```python
from build123d import *

# Parameters (mm, degrees)
SCHIZZO2_W                   = 111.2
SCHIZZO2_H                   = 55
ESTRUSIONE_ESTRUSIONE1_DEPTH = 15
SCHIZZO3_W                   = 14.8
SCHIZZO3_H                   = 55
ESTRUSIONE_ESTRUSIONE2_DEPTH = 24
SCHIZZO4_W                   = 55
SCHIZZO4_H                   = 11.8
ESTRUSIONE_ESTRUSIONE3_DEPTH = 10
SMUSSO1_SIZE                 = 5
SMUSSO2_SIZE                 = 5
FORO_6_0_6_1_D               = 6
SPECCHIA11_COPY_1_D          = 6
SCHIZZO10_R                  = 5.5
TAGLIO_ESTRUSIONE3_DEPTH     = 9
SPECCHIA13_COPY_1_SKETCH_R   = 5.5
SPECCHIA13_COPY_1_DEPTH      = 9
RACCORDO1_R                  = 2
CUT_EXTRUDE1_REACH           = 123.007
SKETCH2_W                    = 27.5
SKETCH2_H                    = 6
SKETCH3_W                    = 111.2
SKETCH3_H                    = 39
BOSS_EXTRUDE1_DEPTH          = 5
SKETCH5_R                    = 15.6
BOSS_EXTRUDE2_DEPTH          = 5.9
FILLET1_R                    = 1
FILLET2_R                    = 5
SCHIZZO11_R                  = 2.9
ESTRUSIONE_ESTRUSIONE4_DEPTH = 5.9
RACCORDO2_R                  = 1
CUT_EXTRUDE2_REACH           = 124.24
SKETCH6_R                    = 2.5
CUT_EXTRUDE3_REACH           = 124.24
SKETCH7_R                    = 2.5
SKETCH8_R                    = 4.5
CUT_EXTRUDE4_DEPTH           = 5
SKETCH9_R                    = 4.5
CUT_EXTRUDE5_DEPTH           = 5


with BuildPart() as part:
    # Schizzo2 → Estrusione-Estrusione1 (new body)
    with BuildSketch(Plane(origin=(0, 0, 0), x_dir=(1, 0, 0), z_dir=(0, 1, 0))):
        Rectangle(SCHIZZO2_W, SCHIZZO2_H)
    extrude(amount=ESTRUSIONE_ESTRUSIONE1_DEPTH)

    # Schizzo3 → Estrusione-Estrusione2 (add)
    with BuildSketch(Plane(origin=(0, 15, 0), x_dir=(1, 0, 0), z_dir=(0, 1, 0))):
        with Locations((48.2, 0)):
            Rectangle(SCHIZZO3_W, SCHIZZO3_H)
    estrusione_estrusione2 = extrude(amount=ESTRUSIONE_ESTRUSIONE2_DEPTH)

    # Schizzo4 → Estrusione-Estrusione3 (add)
    with BuildSketch(Plane.ZY.offset(-40.8)):
        with Locations((0, 33.1)):
            Rectangle(SCHIZZO4_W, SCHIZZO4_H)
    estrusione_estrusione3 = extrude(amount=ESTRUSIONE_ESTRUSIONE3_DEPTH)

    # Smusso1
    smusso1_edges = [part.edges().sort_by_distance(p)[0] for p in [
        (30.8, 33.1, 27.5),
    ]]
    chamfer(smusso1_edges, length=SMUSSO1_SIZE)

    # Specchia2: Estrusione-Estrusione2 across plane
    add(estrusione_estrusione2.mirror(Plane(origin=(0, 0, 0), x_dir=(0, 0, 1), z_dir=(1, 0, 0))))

    # Specchia3: Estrusione-Estrusione3 across plane
    add(estrusione_estrusione3.mirror(Plane(origin=(0, 0, 0), x_dir=(0, 0, 1), z_dir=(1, 0, 0))))

    # Smusso2
    smusso2_edges = [part.edges().sort_by_distance(p)[0] for p in [
        (-30.8, 33.1, 27.5),
    ]]
    chamfer(smusso2_edges, length=SMUSSO2_SIZE)

    # Foro Ø6.0 (6)-1 (through all)
    with Locations(Plane(origin=(0, 15, 0), x_dir=(1, 0, 0), z_dir=(0, 1, 0))):
        with Locations((17.67766953, 17.67766953)):
            foro_6_0_6_1 = Hole(FORO_6_0_6_1_D / 2)

    # Specchia10: Foro Ø6.0 (6)-1 across plane
    add(foro_6_0_6_1.mirror(Plane.XY), mode=Mode.SUBTRACT)

    # Specchia11: Foro Ø6.0 (6)-1 across plane
    add(foro_6_0_6_1.mirror(Plane(origin=(0, 0, 0), x_dir=(0, 0, 1), z_dir=(1, 0, 0))), mode=Mode.SUBTRACT)

    # Specchia11 copy 1 (through all)
    with Locations(Plane(origin=(0, 15, 0), x_dir=(-1, 0, 0), z_dir=(0, 1, 0))):
        with Locations((17.67766953, 17.67766953)):
            Hole(SPECCHIA11_COPY_1_D / 2)

    # Schizzo10 → Taglio-Estrusione3 (cut)
    with BuildSketch(Plane(origin=(0, 15, 0), x_dir=(1, 0, 0), z_dir=(0, 1, 0))):
        with Locations(Location((17.67766953, 17.67766953, 0), (0, 0, 270))):
            Circle(SCHIZZO10_R)
    taglio_estrusione3 = extrude(amount=-TAGLIO_ESTRUSIONE3_DEPTH, mode=Mode.SUBTRACT)

    # Specchia12: Taglio-Estrusione3 across plane
    add(taglio_estrusione3.mirror(Plane.XY), mode=Mode.SUBTRACT)

    # Specchia13: Taglio-Estrusione3 across plane
    add(taglio_estrusione3.mirror(Plane(origin=(0, 0, 0), x_dir=(0, 0, 1), z_dir=(1, 0, 0))), mode=Mode.SUBTRACT)

    # Specchia13 copy 1 sketch → Specchia13 copy 1 (cut)
    with BuildSketch(Plane(origin=(0, 15, 0), x_dir=(-1, 0, 0), z_dir=(0, 1, 0))):
        with Locations(Location((17.67766953, 17.67766953, 0), (0, 0, 270))):
            Circle(SPECCHIA13_COPY_1_SKETCH_R)
    extrude(amount=-SPECCHIA13_COPY_1_DEPTH, mode=Mode.SUBTRACT)

    # Raccordo1
    raccordo1_edges = [part.edges().sort_by_distance(p)[0] for p in [
        (30.8, 27.2, -2.5),
        (30.8, 39, -2.5),
        (-30.8, 27.2, -2.5),
        (-30.8, 39, -2.5),
    ]]
    fillet(raccordo1_edges, radius=RACCORDO1_R)

    # Sketch2 → Cut-Extrude1 (cut, up to next)
    with BuildSketch(Plane.ZY.offset(55.6), mode=Mode.PRIVATE) as cut_extrude1_sk1:
        with Locations((13.75, 18)):
            Rectangle(SKETCH2_W, SKETCH2_H)
    cut_extrude1_tool1 = extrude(cut_extrude1_sk1.sketch, amount=-CUT_EXTRUDE1_REACH, mode=Mode.PRIVATE) & part.part
    add(cut_extrude1_tool1.solids().sort_by_distance((-55.6, 18, 13.75))[0], mode=Mode.SUBTRACT)

    # Sketch3 → Boss-Extrude1 (add)
    with BuildSketch(Plane(origin=(0, 0, -27.5), x_dir=(-1, 0, 0), z_dir=(0, 0, -1))):
        with Locations((0, 19.5)):
            Rectangle(SKETCH3_W, SKETCH3_H)
    extrude(amount=BOSS_EXTRUDE1_DEPTH)

    # Sketch5 → Boss-Extrude2 (add)
    with BuildSketch(Plane.XZ):
        with Locations(Location((0, 0, 0), (0, 0, 270))):
            Circle(SKETCH5_R)
    extrude(amount=BOSS_EXTRUDE2_DEPTH)

    # Fillet1
    fillet1_edges = [part.edges().sort_by_distance(p)[0] for p in [
        (0, -5.9, 15.6),
    ]]
    fillet(fillet1_edges, radius=FILLET1_R)

    # Fillet2
    fillet2_edges = [part.edges().sort_by_distance(p)[0] for p in [
        (-55.6, 7.5, 27.5),
        (55.6, 19.5, -32.5),
        (-55.6, 19.5, -32.5),
        (55.6, 19.5, 27.5),
        (-55.6, 30, 27.5),
    ]]
    fillet(fillet2_edges, radius=FILLET2_R)

    # Schizzo11 → Estrusione-Estrusione4 (add)
    with BuildSketch(Plane.XZ):
        with Locations(Location((0, -25, 0), (0, 0, 270))):
            Circle(SCHIZZO11_R)
        with Locations(Location((-25, 0, 0), (0, 0, 270))):
            Circle(SCHIZZO11_R)
    extrude(amount=ESTRUSIONE_ESTRUSIONE4_DEPTH)

    # Raccordo2
    raccordo2_edges = [part.edges().sort_by_distance(p)[0] for p in [
        (0, -5.9, -22.1),
        (-25, -5.9, 2.9),
    ]]
    fillet(raccordo2_edges, radius=RACCORDO2_R)

    # Sketch6 → Cut-Extrude2 (cut, up to next)
    with BuildSketch(Plane.ZY.offset(55.6), mode=Mode.PRIVATE) as cut_extrude2_sk1:
        with Locations((-12.5, 19.1)):
            Circle(SKETCH6_R)
    cut_extrude2_tool1 = extrude(cut_extrude2_sk1.sketch, amount=-CUT_EXTRUDE2_REACH, mode=Mode.PRIVATE) & part.part
    add(cut_extrude2_tool1.solids().sort_by_distance((-55.6, 19.1, -12.5))[0], mode=Mode.SUBTRACT)

    # Sketch7 → Cut-Extrude3 (cut, up to next)
    with BuildSketch(Plane(origin=(55.6, 0, 0), x_dir=(0, 0, -1), z_dir=(1, 0, 0)), mode=Mode.PRIVATE) as cut_extrude3_sk1:
        with Locations((-12.5, 19.1)):
            Circle(SKETCH7_R)
    cut_extrude3_tool1 = extrude(cut_extrude3_sk1.sketch, amount=-CUT_EXTRUDE3_REACH, mode=Mode.PRIVATE) & part.part
    add(cut_extrude3_tool1.solids().sort_by_distance((55.6, 19.1, 12.5))[0], mode=Mode.SUBTRACT)

    # Sketch8 → Cut-Extrude4 (cut)
    with BuildSketch(Plane.ZY.offset(55.6)):
        with Locations((-12.5, 19.1)):
            Circle(SKETCH8_R)
    extrude(amount=-CUT_EXTRUDE4_DEPTH, mode=Mode.SUBTRACT)

    # Sketch9 → Cut-Extrude5 (cut)
    with BuildSketch(Plane(origin=(55.6, 0, 0), x_dir=(0, 0, -1), z_dir=(1, 0, 0))):
        with Locations((-12.5, 19.1)):
            Circle(SKETCH9_R)
    extrude(amount=-CUT_EXTRUDE5_DEPTH, mode=Mode.SUBTRACT)


solid = part.part
```
Check sheet for the modelled part. Datum: model origin and axes. Units: mm. A direction names the side the tool comes from. Coordinates: 2 decimals unless noted, no trailing zeros. Write each loop counter-clockwise with the first axis right and the second up, starting at its lowest first coordinate (ties: lowest second). Pieces come first, ordered by that corner, then holes. Notation, with made-up numbers: (82, -6.5) -> (108, -6.5) arc R33 cw to (108, 22.5) -> close; hole circle Ø4 at (34, 22.5). An arc over 180 degrees is marked (long way). Use a Markdown table: item, result.
1. Sectioned sample at D-D (z = -25). Enter the section's corners in (x, y).
Reported:
| item | result |
|---|---|
| outline | (-55.6, 0) -> (-2.9, 0) -> (-2.9, -4.9) arc R1 ccw to (-1.9, -5.9) -> (1.9, -5.9) arc R1 ccw to (2.9, -4.9) -> (2.9, 0) -> (55.6, 0) -> (55.6, 39) -> (32.8, 39) arc R2 ccw to (30.8, 37) -> (30.8, 29.2) arc R2 ccw to (32.8, 27.2) -> (40.8, 27.2) -> (40.8, 15) -> (-40.8, 15) -> (-40.8, 27.2) -> (-32.8, 27.2) arc R2 ccw to (-30.8, 29.2) -> (-30.8, 37) arc R2 ccw to (-32.8, 39) -> (-55.6, 39) -> close |
2. Scan lines: line 1 along Z through (x, y) = (18, 9); line 2 along X through (y, z) = (30, 17); line 3 along Y through (x, z) = (-52.15, -12.5). Record each from-to range of solid material in increasing order.
Reported:
| item | result |
|---|---|
| line 1 | z = -32.5 to -23.17, -12.19 to 12.19, 23.17 to 27.5 |
| line 2 | x = -55.6 to -30.8, 30.8 to 55.6 |
| line 3 | y = 0 to 14.6, 23.6 to 39 |
3. Go/stop test with flat-tipped pins: pin 1 Ø12 at (x, z) = (-15.5, 19) entering from +Y; pin 2 Ø6 at (x, z) = (-20, -22) entering from -Y; pin 3 Ø3 at (x, y) = (29.5, 32) entering from +Z; pin 4 Ø5 at (x, z) = (-17.68, -17.68) entering from +Y. Record where each tip stops, or that it passes through.
Reported:
| item | result |
|---|---|
| pin 1 | stops at y = 15 |
| pin 2 | stops at y = 0 |
| pin 3 | stops at z = 22.7 |
| pin 4 | passes through |
4. Sectioned sample at B-B (y = 1.5). Enter the section's corners in (x, z), plus the area to 3 significant figures.
Reported:
| item | result |
|---|---|
| outline | (-55.6, -27.5) arc R5 ccw to (-50.6, -32.5) -> (50.6, -32.5) arc R5 ccw to (55.6, -27.5) -> (55.6, 22.5) arc R5 ccw to (50.6, 27.5) -> (-50.6, 27.5) arc R5 ccw to (-55.6, 22.5) -> close; hole circle Ø6 at (-17.68, -17.68); hole circle Ø6 at (-17.68, 17.68); hole circle Ø6 at (17.68, -17.68); hole circle Ø6 at (17.68, 17.68) |
| area | 6,540 mm2 |
5. Sectioned sample at A-A (z = 19.5). Give the number of separate pieces and of enclosed holes in the cut face, plus the area to 3 significant figures.
Reported:
| item | result |
|---|---|
| separate pieces | 4 |
| enclosed holes | 0 |
| area | 2,280 mm2 |
6. Sectioned sample at C-C (x = 0). Enter the section's corners in (y, z), plus the area to 3 significant figures.
Reported:
| item | result |
|---|---|
| outline | (-5.9, -26.9) arc R1 ccw to (-4.9, -27.9) -> (0, -27.9) -> (0, -32.5) -> (39, -32.5) -> (39, -27.5) -> (15, -27.5) -> (15, 27.5) -> (0, 27.5) -> (0, 15.6) -> (-4.9, 15.6) arc R1 ccw to (-5.9, 14.6) -> (-5.9, -14.6) arc R1 ccw to (-4.9, -15.6) -> (0, -15.6) -> (0, -22.1) -> (-4.9, -22.1) arc R1 ccw to (-5.9, -23.1) -> close |
| area | 1,240 mm2 |
7. Tool access check on faces 1 (the flat face through (-15, 6, -15)), 2 (the flat face through (-33.3, 33, 25)), 3 (the flat face through (-37, 27.2, 0)), 4 (the cylindrical face through (46, 19, 15)). Record the directions out of +Z, -Z, +X, -X, +Y, -Y that give a thin tool (end or side, any length) a straight path to the whole face; none if there is none.
Reported:
| item | result |
|---|---|
| face 1 | +Y |
| face 2 | +Z, +Y |
| face 3 | +Z |
| face 4 | +X |
8. Release check for a two-part mould opening along Y. For faces 5 (the flat face through (-30.8, 33, -3)), 6 (the cylindrical face through (53.135, 20.452, 8.208)), 7 (the flat face through (37, 27.2, 0)), 8 (the flat face through (-15, 6, 15)) record: pulls with the +Y half, pulls with the -Y half, needs draft (parallel to the pull), parting line crosses it, or undercut.
Reported:
| item | result |
|---|---|
| face 5 | needs draft |
| face 6 | undercut |
| face 7 | undercut |
| face 8 | pulls with the +Y half |
